CAD build for the part. Positions are in the model's coordinates, mm. Give positions to 0.01 mm unless a question says otherwise; leave off trailing zeros. Write each loop counter-clockwise with the first axis right and the second up, starting at its lowest first coordinate (ties: lowest second). Pieces come first, ordered by that corner, then holes. Notation, with made-up numbers: (25, 63.5) -> (79, 63.5) arc R12 cw to (79, 81.5) -> close; hole circle Ø11 at (83.25, 79). An arc over 180 degrees is marked (long way). Answer in a Markdown table with one row per item. Add a question column.
```python
from build123d import *

# Parameters (mm, degrees)
SKETCH1_R           = 1.5
BOSS_EXTRUDE1_DEPTH = 47.5
CHAMFER1_SIZE       = 0.15
CUT_EXTRUDE1_START  = -1
SKETCH2_R           = 1.5
SKETCH2_R_2         = 1.25
CUT_EXTRUDE1_DEPTH  = 0.5


with BuildPart() as part:
    # Sketch1 → Boss-Extrude1 (new body)
    with BuildSketch(Plane(origin=(0, 0, 0), x_dir=(1, 0, 0), z_dir=(0, 1, 0))):
        with Locations(Location((0, 0, 0), (0, 0, 270))):
            Circle(SKETCH1_R)
    extrude(amount=BOSS_EXTRUDE1_DEPTH)

    # Chamfer1
    chamfer1_edges = [part.edges().sort_by_distance(p)[0] for p in [
        (0, 0, -1.5),
        (0, 47.5, -1.5),
    ]]
    chamfer(chamfer1_edges, length=CHAMFER1_SIZE)

    # Sketch2 → Cut-Extrude1 (cut)
    with BuildSketch(Plane.XZ.offset(CUT_EXTRUDE1_START)):
        Circle(SKETCH2_R)
        Circle(SKETCH2_R_2, mode=Mode.SUBTRACT)
    extrude(amount=CUT_EXTRUDE1_DEPTH, mode=Mode.SUBTRACT)


solid = part.part
```
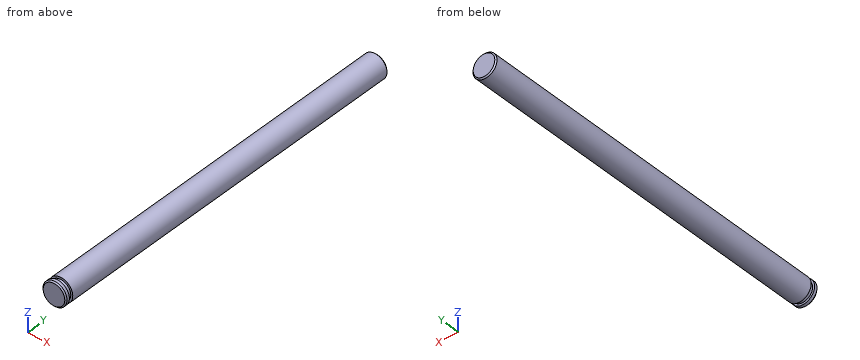
Item 1: Drop a flat-ended pin along its axis: pin 1 Ø1 at (x, y) = (1, 22) entering from -Z. Give the stop position or say it passes through.
Item 2: Probe L1, parallel to Z at x = -0.15, y = 27.5; L2, parallel to Z at x = 0.65, y = 19; L3, parallel to Y at x = 1.2, z = -0.8. List the from-to ranges inside material, lowest first. Write a range as from..to.
Item 3: Slice it at A-A, the plane y = 7.5. List the corners of the cut face in (x, z), then the cut area to 3 significant figures.
Answer key:
| question | item | result |
|---|---|---|
| 1 | pin 1 | stops at z = -1.41 |
| 2 | L1 | z = -1.49..1.49 |
| 2 | L2 | z = -1.35..1.35 |
| 2 | L3 | y = 0.09..0.5, 1..47.41 |
| 3 | outline | circle Ø3 at (0, 0) |
| 3 | area | 7.07 mm² |
